from build123d import *

# Parameters (mm, degrees)
F0_W      = 60
F0_H      = 70
F1_DEPTH  = 18
F2_W      = 2.9
F2_H      = 59
F3_DEPTH  = 13.5
F5_DEPTH  = 16
F7_DEPTH  = 25
F9_DEPTH  = 2
F10_SIZE  = 0.5
F11_R     = 3.45
F11_R_2   = 2.2
F12_DEPTH = 12


with BuildPart() as f1:
    # F0 (on Top) → F1 (new body)
    with BuildSketch(Plane.XY):
        with Locations((30, -35)):
            Rectangle(F0_W, F0_H)
    extrude(amount=F1_DEPTH)

    # F2 (on face) → F3 (cut)
    with BuildSketch(Plane.XY.offset(18)):
        with Locations((46.55, -40.5)):
            Rectangle(F2_W, F2_H)
    extrude(amount=-F3_DEPTH, mode=Mode.SUBTRACT)

    # F4 (on face) → F5 (cut)
    with BuildSketch(Plane.XY.offset(18)):
        with BuildLine():
            Line((4.2371301342, -39.3729269219), (19, -70))
            Line((19, -70), (22.3303290856, -70))
            Line((22.3303290856, -70), (6.8526019079, -37.8898828165))
            ThreePointArc((6.8526019079, -37.8898828165), (12.0206674289, -20.4440960171), (29.8669683324, -23.9900687105))
            Line((29.8669683324, -23.9900687105), (34.880068317, -34.3902538353))
            ThreePointArc((34.880068317, -34.3902538353), (36.2161853291, -36.2452623083), (38.4023255148, -35.5766396993))
            ThreePointArc((38.4023255148, -35.5766396993), (38.6024725197, -35.0710240917), (38.5084373031, -34.5354278406))
            Line((38.5084373031, -34.5354278406), (33.425360506, -23.9900687105))
            ThreePointArc((33.425360506, -23.9900687105), (11.3060254135, -17.4027565566), (4.2371301342, -39.3729269219))
        make_face()
    extrude(amount=-F5_DEPTH, mode=Mode.SUBTRACT)

    # F6 (on face) → F7 (cut)
    with BuildSketch(Plane.XY.offset(18)):
        with BuildLine():
            ThreePointArc((28.5682589784, -33.3296354748), (27.8, -35), (28.5682589784, -36.6703645252))
            ThreePointArc((28.5682589784, -36.6703645252), (30, -37.2), (31.4317410216, -36.6703645252))
            ThreePointArc((31.4317410216, -36.6703645252), (31.9987283767, -35.919284981), (32.2, -35))
            ThreePointArc((32.2, -35), (31.9987283767, -34.080715019), (31.4317410216, -33.3296354748))
            ThreePointArc((31.4317410216, -33.3296354748), (30, -32.8), (28.5682589784, -33.3296354748))
        make_face()
    extrude(amount=-F7_DEPTH, mode=Mode.SUBTRACT)

    # F8 (on face) → F9 (join)
    with BuildSketch(Plane.XY.offset(18)):
        with BuildLine():
            ThreePointArc((8.1348921682, -60.5092924704), (4.6097722286, -60.7804555427), (4.8809353009, -64.3055754823))
            Line((4.8809353009, -64.3055754823), (6.5079137346, -62.4074339763))
            Line((6.5079137346, -62.4074339763), (8.1348921682, -60.5092924704))
        make_face()
        with BuildLine():
            ThreePointArc((55.9920862654, -7.5925660237), (55.7633685117, -6.5479239998), (55.1190646991, -5.6944245177))
            Line((55.1190646991, -5.6944245177), (53.4920862654, -7.5925660237))
            Line((53.4920862654, -7.5925660237), (51.8651078318, -9.4907075296))
            ThreePointArc((51.8651078318, -9.4907075296), (54.5367282893, -9.8638482699), (55.9920862654, -7.5925660237))
        make_face()
        with BuildLine():
            Line((6.5079137346, -62.4074339763), (4.8809353009, -64.3055754823))
            ThreePointArc((4.8809353009, -64.3055754823), (7.5525557584, -64.6787162226), (9.0079137346, -62.4074339763))
            ThreePointArc((9.0079137346, -62.4074339763), (8.7791959808, -61.3627919525), (8.1348921682, -60.5092924704))
            Line((8.1348921682, -60.5092924704), (6.5079137346, -62.4074339763))
        make_face()
        with BuildLine():
            Line((53.4920862654, -7.5925660237), (55.1190646991, -5.6944245177))
            ThreePointArc((55.1190646991, -5.6944245177), (51.5939447595, -5.96558759), (51.8651078318, -9.4907075296))
            Line((51.8651078318, -9.4907075296), (53.4920862654, -7.5925660237))
        make_face()
    extrude(amount=F9_DEPTH)

    # F10
    f10_edges = [f1.edges().sort_by_distance(p)[0] for p in [
        (8.134892, -60.509292, 20),
        (51.865108, -9.490708, 20),
        (27.8, -35, 18),
    ]]
    chamfer(f10_edges, length=F10_SIZE)

    # F11 (on face) → F12 (cut)
    with BuildSketch(Plane(origin=(0, 0, 0), x_dir=(1, 0, 0), z_dir=(0, 0, -1))):
        with Locations((30, 35)):
            Circle(F11_R)
        with Locations((30, 35)):
            Circle(F11_R_2, mode=Mode.SUBTRACT)
    extrude(amount=-F12_DEPTH, mode=Mode.SUBTRACT)


solid = f1.part
Work out the finished part from the listing and answer in its coordinate system (mm). A direction names the side the tool comes from. Coordinates: 2 decimals unless noted, no trailing zeros. Order: outer loops, then holes, each group sorted by start corner. A loop starts at its lowest first (then second) coordinate and runs counter-clockwise, first axis right, second up. Notation, with made-up numbers: (19.25, -0.5) - (74.25, -0.5) arc R17 cw to (74.25, 19.5) - close; hole circle Ø8 at (13, 13.25). An arc over 180 degrees is marked (long way). Put each result on its own line as item: value. Start each with the question number.
1) Find section C-C (y = -22). Give the vertices of the cut face in (x, z).
2) Flat-ended cylindrical pins translate along their axes: pin 1 (18 mm diameter, centred on x = 17, y = -45.5, fed in from +Z); pin 2 (0.9 mm diameter, centred on x = 46.5, z = 13, fed in from -Y). Find the tip coordinate at first contact, or state that the pin passes through.
3) Find section B-B (x = 12.5). Give the vertices of the cut face in (y, z).
4) For a pull along X with two mould halves and no side action, classify faces 1 (the flat face through (60, -35, 9)), 2 (the flat face through (53, -8, 20)), 3 (the cylindrical face through (27.262, -32.901, 5.916)) as released by +X, released by -X, zero draft, split by the parting line, or undercut.
5) Find the intervals of material crossed by line 1 (X direction, y = -14, z = 13); line 2 (X direction, y = -46, z = 5.5); line 3 (X direction, y = -35, z = 7), in increasing order. Write a range as from..to.
6) Find section A-A (z = 13). Give the vertices of the cut face in (x, y), plus the area to 3 significant figures.
7) For faces 4 (the flat face through (23, -35, 0)), 5 (the flat face through (32.34, -29.12, 10.11)), 6 (the flat face through (30, 0, 9)), 7 (the flat face through (30.7, -32.7, 12)), 8 (the flat face through (45.1, -41, 11)), determine the directions among +Z, -Z, +X, -X, +Y, -Y from which every point of the face is accessible in a straight line to the end or side of a thin tool.
8) Find section D-D (z = 3.5). Give the vertices of the cut face in (x, y).
Results list:
1. outline: (0, 0) - (60, 0) - (60, 18) - (48, 18) - (48, 4.5) - (45.1, 4.5) - (45.1, 18) - (32.12, 18) - (32.12, 2) - (28.07, 2) - (28.07, 18) - (9.93, 18) - (9.93, 2) - (5.87, 2) - (5.87, 18) - (0, 18) - close
2. pin 1: stops at z = 18
2. pin 2: stops at y = -11
3. outline: (-70, 0) - (0, 0) - (0, 18) - (-16.83, 18) - (-16.83, 2) - (-20.17, 2) - (-20.17, 18) - (-49.61, 18) - (-49.61, 2) - (-56.52, 2) - (-56.52, 18) - (-70, 18) - close
4. face 1: released by +X
4. face 2: zero draft
4. face 3: undercut
5. line 1: x = 0..45.1, 48..60
5. line 2: x = 0..7.43, 10.76..45.1, 48..60
5. line 3: x = 0..2.77, 5.84..26.55, 33.45..34.98, 38.61..45.1, 48..60
6. outline: (0, -70) - (19, -70) - (4.24, -39.37) arc R16.5 cw to (33.43, -23.99) - (38.51, -34.54) arc R1 cw to (38.4, -35.58) arc R1.96 cw to (34.88, -34.39) - (29.87, -23.99) arc R13.5 ccw to (6.85, -37.89) - (22.33, -70) - (45.1, -70) - (45.1, -11) - (48, -11) - (48, -70) - (60, -70) - (60, 0) - (0, 0) - close; hole circle Ø4.4 at (30, -35)
6. area: 3,730 mm^2
7. face 4: -Z, +X, -X, +Y, -Y
7. face 5: +Z
7. face 6: +Z, -Z, +X, -X, +Y
7. face 7: -Z
7. face 8: +Z, -Y
8. outline: (0, -70) - (19, -70) - (4.24, -39.37) arc R16.5 cw to (33.43, -23.99) - (38.51, -34.54) arc R1 cw to (38.4, -35.58) arc R1.96 cw to (34.88, -34.39) - (29.87, -23.99) arc R13.5 ccw to (6.85, -37.89) - (22.33, -70) - (60, -70) - (60, 0) - (0, 0) - close; hole circle Ø6.9 at (30, -35)
